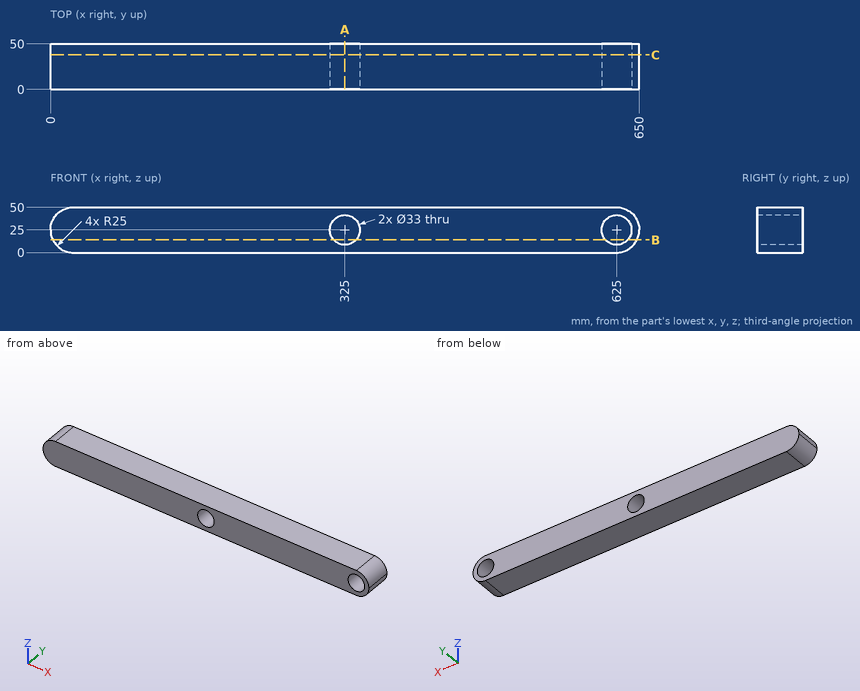
Study the drawing (mm; zero at the part's minimum x, y, z) and answer. Give positions to 0.01 mm unless a question says otherwise; leave off trailing zeros. Write each loop counter-clockwise with the first axis right and the second up, starting at its lowest first coordinate (ties: lowest second). Pieces come first, ordered by that corner, then holes. Notation, with made-up numbers: (23, 39) -> (41, 39) arc R21 ccw to (41, 72) -> close; hole circle Ø10 at (41.25, 70). An arc over 180 degrees is marked (long way). Write item = value, one per line. Start each with the question number.
1) The part is cut by section C-C, the plane y = 38. Count the separate pieces of the cut face and the enclosed holes in it, and give its area (3 significant figures).
2) Straight lines are drawn through the part: line 1 along X through (y, z) = (16, 25); line 2 along X through (y, z) = (35.5, 21.5); line 3 along Z through (x, y) = (324, 14.5). For each, find the intervals that lie inside material, in ascending order.
3) Each of these flat-tipped pins is pushed along its axis until it touches: pin 1 (10 mm diameter, centred on x = 77.5, y = 30, fed in from -Z); pin 2 (2 mm diameter, centred on y = 35, z = 14.5, fed in from -X). Where does it stop, or does it pass through?
4) The part is cut by section B-B, the plane z = 14. Determine the outline of the cut face in (x, y).
5) The part is cut by section A-A, the plane x = 325. Determine the outline of the cut face in (y, z).
Solutions:
q1.separate_pieces = 1
q1.enclosed_holes = 2
q1.area = 30,300 mm²
q2.line_1 = 0 to 308.5, 341.5 to 608.5, 641.5 to 650
q2.line_2 = 0.25 to 308.88, 341.12 to 608.88, 641.12 to 649.75
q2.line_3 = 0 to 8.53, 41.47 to 50
q3.pin_1 = 0
q3.pin_2 = 1.88
q4.outline = (2.55, 0) -> (312.7, 0) -> (312.7, 50) -> (2.55, 50) -> close; (337.3, 0) -> (612.7, 0) -> (612.7, 50) -> (337.3, 50) -> close; (637.3, 0) -> (647.45, 0) -> (647.45, 50) -> (637.3, 50) -> close
q5.outline = (0, 0) -> (50, 0) -> (50, 8.5) -> (0, 8.5) -> close; (0, 41.5) -> (50, 41.5) -> (50, 50) -> (0, 50) -> close
